Verification items for this drawing (mm, ordinates from the low corner). A direction names the side the tool comes from. Give positions to 0.01 mm unless a question says otherwise; leave off trailing zeros. Order: outer loops, then holes, each group sorted by start corner. A loop starts at its lowest first (then second) coordinate and runs counter-clockwise, first axis right, second up. Notation, with made-up numbers: (61, -30.5) - (88, -30.5) arc R29 ccw to (88, -0.5) - close; hole circle Ø1 at (21.25, -20.75). An arc over 180 degrees is marked (long way). Put each result on its own line as item: value. Start each with the question number.
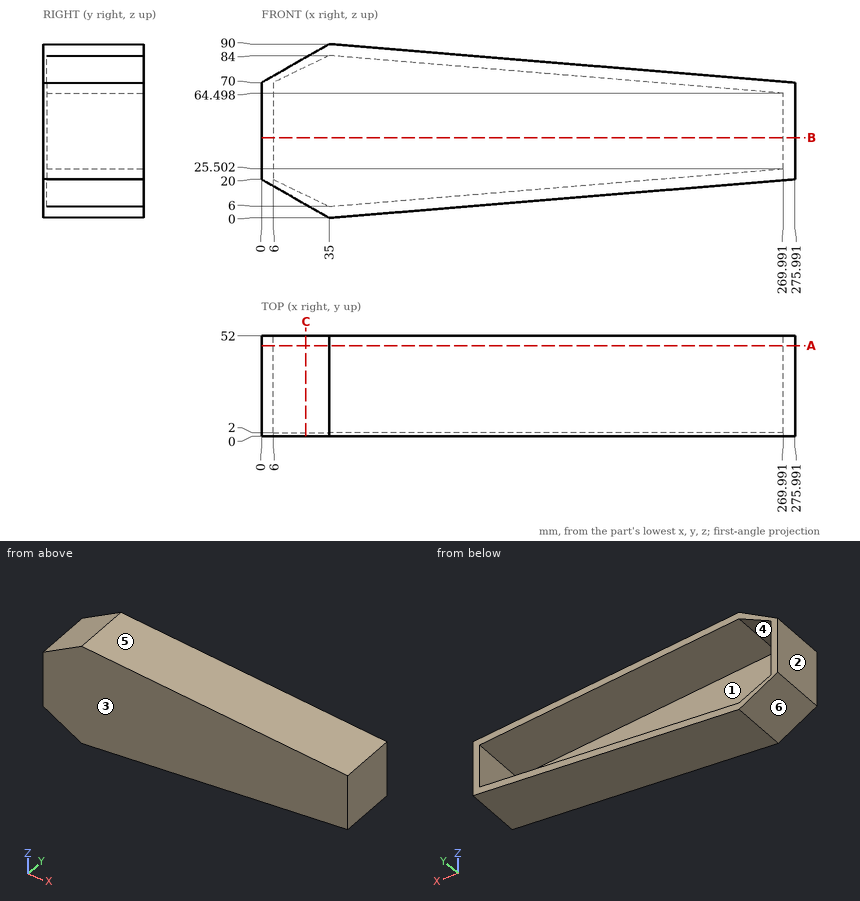
Item 1: Cross-section at A-A (y = 47). Enter the section's corners in (x, z).
Item 2: Thickness scan on line 1 along X through (y, z) = (6, 46.5); line 2 along Y through (x, z) = (258, 53.5); line 3 along Z through (x, y) = (240, 25). Record the ranges inside material, lowest first.
Item 3: Set-up check for the marked faces 1 and 2: record each of +Z, -Z, +X, -X, +Y, -Y from which the full face is reachable in a straight line by a thin tool's end or side.
Item 4: Cross-section at B-B (z = 41.5). Enter the section's corners in (x, y), and give its area (3 significant figures).
Item 5: Cross-section at C-C (x = 23). Enter the section's corners in (y, z).
Item 6: Gauge pin test, flat ends, axial feed: pin 1 Ø12 at (y, z) = (12.5, 60) entering from -X; pin 2 Ø3 at (x, y) = (186, 20) entering from +Z; pin 3 Ø10 at (y, z) = (17, 79) entering from -X; pin 4 Ø5 at (x, y) = (222.5, 23) entering from -Z. Record the tip position at first contact, or that the pin passes through.
Item 7: Release check for a two-part mould opening along X. For the marked faces 3, 4, 5 and 6 record: +X half, -X half, draft (parallel to the pull), parting line (faces both ways), or undercut.
Recorded:
1. outline: (0, 20) - (35, 0) - (275.99, 20) - (275.99, 70) - (35, 90) - (0, 70) - close; hole (6, 20) - (35, 6) - (269.99, 25.5) - (269.99, 64.5) - (35, 84) - (6, 70) - close
2. line 1: x = 0 to 6, 269.99 to 275.99
2. line 2: y = 0 to 2
2. line 3: z = 17.01 to 23.01, 66.99 to 72.99
3. face 1: +Y
3. face 2: +Z, -Z, -X, +Y, -Y
4. outline: (0, 0) - (275.99, 0) - (275.99, 52) - (269.99, 52) - (269.99, 2) - (6, 2) - (6, 52) - (0, 52) - close
4. area: 1,150 mm^2
5. outline: (0, 6.86) - (52, 6.86) - (52, 11.79) - (2, 11.79) - (2, 78.21) - (52, 78.21) - (52, 83.14) - (0, 83.14) - close
6. pin 1: stops at x = 0
6. pin 2: stops at z = 77.59
6. pin 3: stops at x = 7
6. pin 4: stops at z = 15.35
7. face 3: draft
7. face 4: undercut
7. face 5: +X half
7. face 6: -X half
